```python
from build123d import *

# Parameters (mm, degrees)
F0_W      = 127
F0_H      = 76.2
F1_DEPTH  = 34.036
F2_R      = 5
F3_W      = 13.8
F3_H      = 6.427399
F4_DEPTH  = 16.44
F5_W      = 13.640474
F5_H      = 6.40964
F6_DEPTH  = 16.44
F7_R      = 1.750354
F8_DEPTH  = 2
F9_R      = 1.747334
F10_DEPTH = 2
F11_R     = 1.782864
F12_DEPTH = 2
F13_R     = 1.715202
F14_DEPTH = 2
F15_W     = 1.989198
F15_H     = 3.315331
F16_DEPTH = 2
F17_W     = 9.945992
F17_H     = 4.199421
F18_DEPTH = 1.5


with BuildPart() as f1:
    # F0 (on Front) → F1 (new body)
    with BuildSketch(Plane.XZ):
        Rectangle(F0_W, F0_H)
    extrude(amount=F1_DEPTH)

    # F2
    f2_edges = [f1.edges().sort_by_distance(p)[0] for p in [
        (0, -34.036, 38.1),
        (0, 0, 38.1),
        (0, -34.036, -38.1),
        (0, 0, -38.1),
    ]]
    fillet(f2_edges, radius=F2_R)

    # F3 (on face) → F4 (cut)
    with BuildSketch(Plane.YZ.offset(63.5)):
        with Locations((-17.902091, 22.212722)):
            Rectangle(F3_W, F3_H)
    extrude(amount=-F4_DEPTH, mode=Mode.SUBTRACT)

    # F5 (on face) → F6 (cut)
    with BuildSketch(Plane.YZ.offset(63.5)):
        with Locations((-17.981854, 8.840884)):
            Rectangle(F5_W, F5_H)
    extrude(amount=-F6_DEPTH, mode=Mode.SUBTRACT)

    # F7 (on face) → F8 (cut)
    with BuildSketch(Plane.YZ.offset(63.5)):
        with Locations((-29.259426, -7.352235)):
            Circle(F7_R)
    extrude(amount=-F8_DEPTH, mode=Mode.SUBTRACT)

    # F9 (on face) → F10 (cut)
    with BuildSketch(Plane.YZ.offset(63.5)):
        with Locations((-21.881189, -7.29373)):
            Circle(F9_R)
    extrude(amount=-F10_DEPTH, mode=Mode.SUBTRACT)

    # F11 (on face) → F12 (cut)
    with BuildSketch(Plane.YZ.offset(63.5)):
        with Locations((-14.947511, -7.233127)):
            Circle(F11_R)
    extrude(amount=-F12_DEPTH, mode=Mode.SUBTRACT)

    # F13 (on face) → F14 (cut)
    with BuildSketch(Plane.YZ.offset(63.5)):
        with Locations((-8.288329, -7.326883)):
            Circle(F13_R)
    extrude(amount=-F14_DEPTH, mode=Mode.SUBTRACT)

    # F15 (on face) → F16 (cut)
    with BuildSketch(Plane.YZ.offset(63.5)):
        with Locations((-18.123812, -23.649363)):
            Rectangle(F15_W, F15_H)
    extrude(amount=-F16_DEPTH, mode=Mode.SUBTRACT)

    # F17 (on face) → F18 (join)
    with BuildSketch(Plane.XY.offset(38.1)):
        with Locations((54.813484, -21.439144)):
            Rectangle(F17_W, F17_H)
    extrude(amount=F18_DEPTH)


solid = f1.part
```
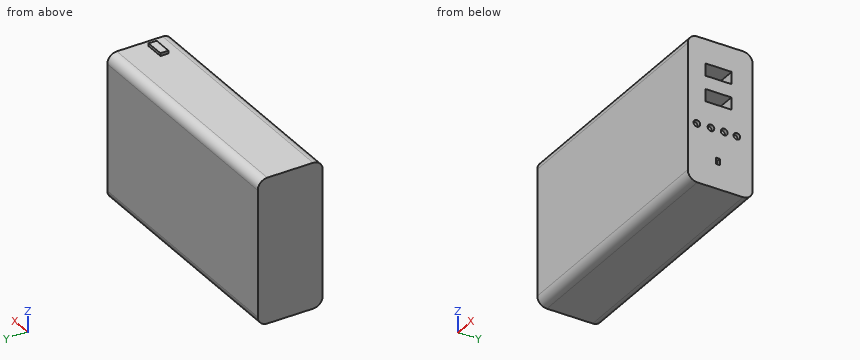
Model file for the job. Use its own axes, mm. Give positions to 0.01 mm unless a question says otherwise; leave off trailing zeros. Write each loop counter-clockwise with the first axis right and the second up, starting at its lowest first coordinate (ties: lowest second). Pieces come first, ordered by that corner, then holes. Notation, with made-up numbers: (64, 54.25) -> (120, 54.25) arc R10 cw to (120, 59.25) -> close; hole circle Ø8 at (-16.5, 53). An arc over 180 degrees is marked (long way). Use CSV: the item, a comma, the result in double quotes. Start each with the question number.
1) Drill centre lines: L1, parallel to Z at x = 57.5, y = -13; L2, parallel to Z at x = -30.5, y = -6; L3, parallel to X at y = -11.5, z = 12. Where is each one in solid material? Low to high.
2) Cut at B-B on z = 24. List the corners of the cut face in (x, y).
3) Cut at C-C on x = 13. List the corners of the cut face in (y, z).
4) Cut at A-A on x = 53. List the corners of the cut face in (y, z), plus the area to 3 significant figures.
5) Pin check, flat tips, straight feed: P1, Ø3, axis at y = -14.5, z = -7, coming from the +X side; P2, Ø1, axis at x = -27, y = -25, coming from the +Z side; P3, Ø3, axis at y = -19, z = 8.5, coming from the +X side; P4, Ø1, axis at y = -18, z = -23, coming from the +X side. Stop position of each tip, or through.
Final values:
1,L1,"z = -38.1 to 5.64, 12.05 to 19, 25.43 to 38.1"
1,L2,"z = -38.1 to 38.1"
1,L3,"x = -63.5 to 47.06"
2,outline,"(-63.5, -34.04) -> (63.5, -34.04) -> (63.5, -24.8) -> (47.06, -24.8) -> (47.06, -11) -> (63.5, -11) -> (63.5, 0) -> (-63.5, 0) -> close"
3,outline,"(-34.04, -33.1) arc R5 ccw to (-29.04, -38.1) -> (-5, -38.1) arc R5 ccw to (0, -33.1) -> (0, 33.1) arc R5 ccw to (-5, 38.1) -> (-29.04, 38.1) arc R5 ccw to (-34.04, 33.1) -> close"
4,outline,"(-34.04, -33.1) arc R5 ccw to (-29.04, -38.1) -> (-5, -38.1) arc R5 ccw to (0, -33.1) -> (0, 33.1) arc R5 ccw to (-5, 38.1) -> (-19.34, 38.1) -> (-19.34, 39.6) -> (-23.54, 39.6) -> (-23.54, 38.1) -> (-29.04, 38.1) arc R5 ccw to (-34.04, 33.1) -> close; hole (-24.8, 5.64) -> (-11.16, 5.64) -> (-11.16, 12.05) -> (-24.8, 12.05) -> close; hole (-24.8, 19) -> (-11, 19) -> (-11, 25.43) -> (-24.8, 25.43) -> close"
4,area,"2,400 mm2"
5,P1,"stops at x = 63.5"
5,P2,"stops at z = 38.1"
5,P3,"stops at x = 47.06"
5,P4,"stops at x = 61.5"
